Build history of the part. All positions in model axes, mm. A direction names the side the tool comes from. Give positions to 0.01 mm unless a question says otherwise; leave off trailing zeros. Order: outer loops, then holes, each group sorted by start corner. A loop starts at its lowest first (then second) coordinate and runs counter-clockwise, first axis right, second up. Notation, with made-up numbers: (-8.75, 2) - (35.25, 2) arc R12 cw to (35.25, 8) - close; hole circle Ø10 at (59, 83.5). An arc over 180 degrees is marked (long way). Use a Markdown table: item, result. Add a question column.
(1) Flat gauge pins, fed straight in: pin 1 (12 mm diameter, centred on x = 4.5, y = 38, fed in from +Z); pin 2 (10.5 mm diameter, centred on y = 62, z = -2.5, fed in from +X); pin 3 (10 mm diameter, centred on y = 30.5, z = 6.5, fed in from -X). Where does each tip first touch, or does it go through?
(2) Mould opens along Z. For faces 1 (the face through (72, 41, -6.15)), 2 (the face through (-72.12, 79.33, 9.8)), 3 (the face through (84.646, 44, 7)) say: +Z half, -Z half, draft (parallel to the pull), parting line (faces both ways), or undercut.
(3) Slice it at B-B (x = -62). Write the cut outline in (y, z).
(4) Slice it at C-C (y = 31.5). Write the cut outline in (x, z), then the cut area to 3 significant figures.
(5) Wall check: line 1 (Y direction, x = -77.25, z = 0); line 2 (X direction, y = 57.5, z = -3.5); line 3 (Z direction, x = -68.5, y = 30). Give the ranges that are in metal, low to high.
(6) Slice it at A-A (y = 65). Write the cut outline in (x, z), then the cut area to 3 significant figures.
(7) Which spindle directions (+Z, -Z, +X, -X, +Y, -Y) get a long thin tool onto all of the face, cutting with end or side? Do faces 4 (the face through (-72, 41, 6.15)), 5 (the face through (72, 52.05, 0)), 6 (the face through (-55.426, 9.972, -0.144)), 7 (the face through (-84.646, 44, 7)), 8 (the face through (-1, 3, 50.8)). Say none if no direction does.
(8) Slice it at D-D (x = 6.5). Write the cut outline in (y, z).
from build123d import *

# Parameters (mm, degrees)
SKETCH1_W           = 177.8
SKETCH1_H           = 101.6
BOSS_EXTRUDE1_DEPTH = 6.35
BOSS_EXTRUDE2_DEPTH = 177.8
SKETCH3_W           = 57.658
SKETCH3_H           = 101.6
SKETCH3_W_2         = 4.2545
CUT_EXTRUDE1_DEPTH  = 129.722963579
FILLET1_R           = 43.18
FILLET2_R           = 12.7
FILLET3_R           = 2.286
SKETCH5_R           = 1
SKETCH5_W           = 12.3
SKETCH5_H           = 22.7
CUT_EXTRUDE2_DEPTH  = 178.330785165
CUT_EXTRUDE3_START  = 118.491
SKETCH5_2_R         = 1
SKETCH5_2_W         = 12.3
SKETCH5_2_H         = 22.7
CUT_EXTRUDE3_DEPTH  = 59.839785165


with BuildPart() as part:
    # Sketch1 → Boss-Extrude1 (new body)
    with BuildSketch(Plane(origin=(0, 0, 0), x_dir=(1, 0, 0), z_dir=(0, 1, 0))):
        Rectangle(SKETCH1_W, SKETCH1_H)
    extrude(amount=BOSS_EXTRUDE1_DEPTH)

    # Sketch2 → Boss-Extrude2 (add)
    with BuildSketch(Plane.ZY.offset(88.9)):
        with BuildLine():
            Line((0, 69.088), (0, 6.35))
            Line((0, 6.35), (10.287, 6.35))
            Line((10.287, 6.35), (10.287, 76.2))
            ThreePointArc((10.287, 76.2), (9.226129892, 80.749823756), (6.26232882, 84.361225812))
            Line((6.26232882, 84.361225812), (4.329511283, 81.842328956))
            ThreePointArc((4.329511283, 81.842328956), (6.734567081, 73.913922523), (0, 69.088))
        make_face()
        with BuildLine():
            Line((-10.287, 76.2), (-10.287, 6.35))
            Line((-10.287, 6.35), (0, 6.35))
            Line((0, 6.35), (0, 69.088))
            ThreePointArc((0, 69.088), (-6.734567081, 73.913922523), (-4.329511283, 81.842328956))
            Line((-4.329511283, 81.842328956), (-6.26232882, 84.361225812))
            ThreePointArc((-6.26232882, 84.361225812), (-9.226129892, 80.749823756), (-10.287, 76.2))
        make_face()
    extrude(amount=-BOSS_EXTRUDE2_DEPTH)

    # Sketch3 → Cut-Extrude1 (cut, through all)
    with BuildSketch(Plane(origin=(0, 6.35, 0), x_dir=(1, 0, 0), z_dir=(0, 1, 0))):
        with Locations((-30.4165, 0)):
            Rectangle(SKETCH3_W, SKETCH3_H)
        with Locations((30.4165, 0)):
            Rectangle(SKETCH3_W, SKETCH3_H)
        with Locations((86.77275, 0)):
            Rectangle(SKETCH3_W_2, SKETCH3_H)
        with Locations((-86.77275, 0)):
            Rectangle(SKETCH3_W_2, SKETCH3_H)
    extrude(amount=CUT_EXTRUDE1_DEPTH, mode=Mode.SUBTRACT)

    # Fillet1
    fillet1_edges = [part.edges().sort_by_distance(p)[0] for p in [
        (1.5875, 6.35, 0),
        (-1.5875, 6.35, 0),
    ]]
    fillet(fillet1_edges, radius=FILLET1_R)

    # Fillet2
    fillet2_edges = [part.edges().sort_by_distance(p)[0] for p in [
        (59.2455, 6.35, 0),
        (-59.2455, 6.35, 0),
    ]]
    fillet(fillet2_edges, radius=FILLET2_R)

    # Fillet3
    fillet3_edges = [part.edges().sort_by_distance(p)[0] for p in [
        (71.9455, 84.361225812, -6.26232882),
        (0, 84.361225812, -6.26232882),
        (-71.9455, 84.361225812, -6.26232882),
        (71.9455, 84.361225812, 6.26232882),
        (0, 84.361225812, 6.26232882),
        (-71.9455, 84.361225812, 6.26232882),
    ]]
    fillet(fillet3_edges, radius=FILLET3_R)

    # Sketch5 → Cut-Extrude2 (cut, through all)
    with BuildSketch(Plane.ZY.offset(-59.2455)):
        with Locations((0, 54.7)):
            Circle(SKETCH5_R)
        with Locations((0, 26.7)):
            Circle(SKETCH5_R)
        with Locations((0, 40.7)):
            Rectangle(SKETCH5_W, SKETCH5_H)
    extrude(amount=-CUT_EXTRUDE2_DEPTH, mode=Mode.SUBTRACT)

    # Sketch5<2> → Cut-Extrude3 (cut, through all)
    with BuildSketch(Plane.ZY.offset(-59.2455).offset(CUT_EXTRUDE3_START)):
        with Locations((0, 54.7)):
            Circle(SKETCH5_2_R)
        with Locations((0, 26.7)):
            Circle(SKETCH5_2_R)
        with Locations((0, 40.7)):
            Rectangle(SKETCH5_2_W, SKETCH5_2_H)
    extrude(amount=CUT_EXTRUDE3_DEPTH, mode=Mode.SUBTRACT)


solid = part.part
Solution:
| question | item | result |
|---|---|---|
| 1 | pin 1 | z = 10.29 |
| 1 | pin 2 | x = 84.65 |
| 1 | pin 3 | x = -84.65 |
| 2 | face 1 | undercut |
| 2 | face 2 | +Z half |
| 2 | face 3 | draft |
| 3 | outline | (0, -50.8) - (6.35, -50.8) - (6.35, -10.29) - (76.2, -10.29) arc R10.29 ccw to (82.23, -8.33) arc R2.29 ccw to (82.28, -4.67) - (81.84, -4.33) arc R7.11 cw (long way) to (81.84, 4.33) - (82.28, 4.67) arc R2.29 ccw to (82.23, 8.33) arc R10.29 ccw to (76.2, 10.29) - (6.35, 10.29) - (6.35, 50.8) - (0, 50.8) - close; hole circle Ø2 at (26.7, 0); hole (29.35, -6.15) - (52.05, -6.15) - (52.05, 6.15) - (29.35, 6.15) - close; hole circle Ø2 at (54.7, 0) |
| 4 | outline | (-84.65, -10.29) - (-59.25, -10.29) - (-59.25, -6.15) - (-84.65, -6.15) - close; (-84.65, 6.15) - (-59.25, 6.15) - (-59.25, 10.29) - (-84.65, 10.29) - close; (-5.53, -10.29) - (5.53, -10.29) - (5.53, 10.29) - (-5.53, 10.29) - close; (59.25, -10.29) - (84.65, -10.29) - (84.65, -6.15) - (59.25, -6.15) - close; (59.25, 6.15) - (84.65, 6.15) - (84.65, 10.29) - (59.25, 10.29) - close |
| 4 | area | 648 mm2 |
| 5 | line 1 | 0 to 25.7, 27.7 to 29.35, 52.05 to 53.7, 55.7 to 69.09 |
| 5 | line 2 | -84.65 to -59.25, -1.59 to 1.59, 59.25 to 84.65 |
| 5 | line 3 | -10.29 to -6.15, 6.15 to 10.29 |
| 6 | outline | (-84.65, -10.29) - (-59.25, -10.29) - (-59.25, 10.29) - (-84.65, 10.29) - close; (-1.59, -10.29) - (1.59, -10.29) - (1.59, 10.29) - (-1.59, 10.29) - close; (59.25, -10.29) - (84.65, -10.29) - (84.65, 10.29) - (59.25, 10.29) - close |
| 6 | area | 1,110 mm2 |
| 7 | face 4 | -X |
| 7 | face 5 | +X |
| 7 | face 6 | +Z, -Z, +Y |
| 7 | face 7 | +Z, -Z, -X, +Y |
| 7 | face 8 | +Z, +X, -X, +Y, -Y |
| 8 | outline | (0, -50.8) - (6.35, -50.8) - (6.35, -10.29) - (29.53, -10.29) - (29.53, 10.29) - (6.35, 10.29) - (6.35, 50.8) - (0, 50.8) - close |
